For this review, use the dimensioned drawing (mm, ordinates from the lowest corner) and the shaded views. Give positions to 0.01 mm unless a question says otherwise; leave off trailing zeros. Order: outer loops, then holes, each group sorted by start corner. A loop starts at its lowest first (then second) coordinate and runs counter-clockwise, first axis right, second up.
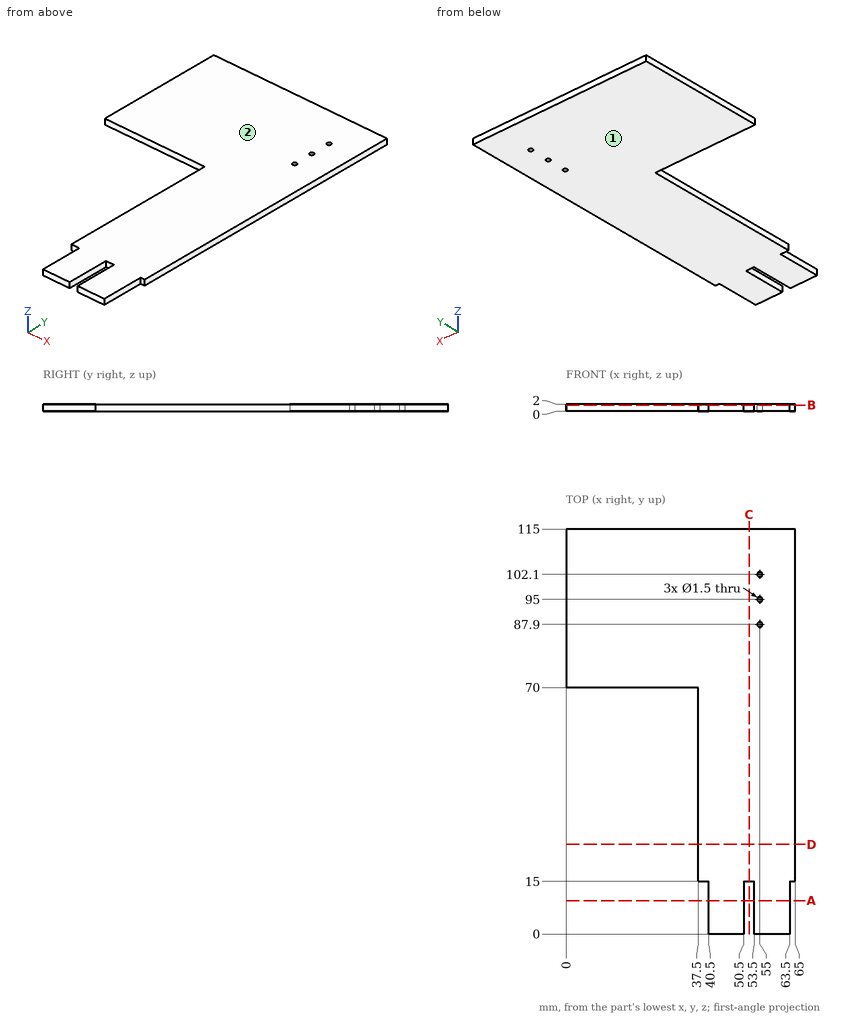
1. For line 1 along Y through (x, z) = (55, 0.5); line 2 along X through (y, z) = (95, 1.4); line 3 along X through (y, z) = (30, 0.75), list the stretches that pass through material, from the lowest coordinate up.
Recorded:
line 1: y = 0 to 87.15, 88.65 to 94.25, 95.75 to 101.35, 102.85 to 115
line 2: x = 0 to 54.25, 55.75 to 65
line 3: x = 37.5 to 65
2. Take a section at D-D (y = 25.5). State the section outline as (x, z) points.
Recorded:
outline: (37.5, 0) - (65, 0) - (65, 2) - (37.5, 2) - close
3. Take a section at B-B (z = 1.65). State the section outline as (x, y) points.
Recorded:
outline: (0, 70) - (37.5, 70) - (37.5, 15) - (40.5, 15) - (40.5, 0) - (50.5, 0) - (50.5, 15) - (53.5, 15) - (53.5, 0) - (63.5, 0) - (63.5, 15) - (65, 15) - (65, 115) - (0, 115) - close; hole circle Ø1.5 at (55, 87.9); hole circle Ø1.5 at (55, 95); hole circle Ø1.5 at (55, 102.1)
4. Take a section at A-A (y = 9.5). State the section outline as (x, z) points.
Recorded:
outline: (40.5, 0) - (50.5, 0) - (50.5, 2) - (40.5, 2) - close; (53.5, 0) - (63.5, 0) - (63.5, 2) - (53.5, 2) - close
5. Take a section at C-C (x = 52). State the section outline as (y, z) points, then the cut area to 3 significant figures.
Recorded:
outline: (15, 0) - (115, 0) - (115, 2) - (15, 2) - close
area: 200 mm2
6. Draft analysis for pull direction Z (two halves, no side actions). For the marked faces 1 and 2, state which applies: pulls with the +Z half, pulls with the -Z half, needs draft (parallel to the pull), parting line crosses it, or undercut.
Recorded:
face 1: pulls with the -Z half
face 2: pulls with the +Z half
7. For pin 1 (1.2 mm diameter, centred on x = 55, y = 95, fed in from -Z) (3 decimals); pin 2 (1 mm diameter, centred on y = 36, z = 1, fed in from -X); pin 3 (1 mm diameter, centred on y = 7.5, z = 1, fed in from -X), all flat-tipped, find the tip position at first contact; note any pin that passes through.
Recorded:
pin 1: passes through
pin 2: stops at x = 37.5
pin 3: stops at x = 40.5
